Read the model definition and answer for the solid it produces. Units are mm, in the model's axes. Face numbers are marked on the shaded views. Coordinates: 2 decimals unless noted, no trailing zeros. Order: outer loops, then holes, each group sorted by start corner. A loop starts at its lowest first (then second) coordinate and runs counter-clockwise, first axis right, second up. Notation, with made-up numbers: (3, 75) -> (24, 75) arc R17 cw to (24, 105) -> close; hole circle Ø11 at (-39, 19). An arc over 180 degrees is marked (long way). Answer as a JSON object with one key per item and string values. Group by question number.
1) Section A-A on x = -48.75 is taken. Determine the outline of the cut face in (y, z).
2) Given pin 1 (1.5 mm diameter, centred on x = -51.5, y = 25.5, fed in from +Z); pin 2 (1.1 mm diameter, centred on y = 27.5, z = 3, fed in from +X); pin 3 (2 mm diameter, centred on y = 28, z = 4.5, fed in from -X), each flat-ended and moving along its own axis, determine where each tip first touches the part or whether it passes through.
3) Determine the mould class of the marked faces 1, 2, 3 and 4 for opening direction X: released by +X, released by -X, zero draft, split by the parting line, or undercut.
4) Consider L1, parallel to X at y = 26.75, z = 2.85; L2, parallel to Z at x = -50, y = 29.5; L3, parallel to X at y = 27.25, z = 0.9. Determine where each line is inside the solid, lowest interval first.
5) Section C-C on z = 3.15 is taken. Determine the outline of the cut face in (x, y), and give its area (3 significant figures).
6) Section D-D on x = -50 is taken. Determine the outline of the cut face in (y, z), and give its area (3 significant figures).
7) Section B-B on y = 24.75 is taken. Determine the outline of the cut face in (x, z).
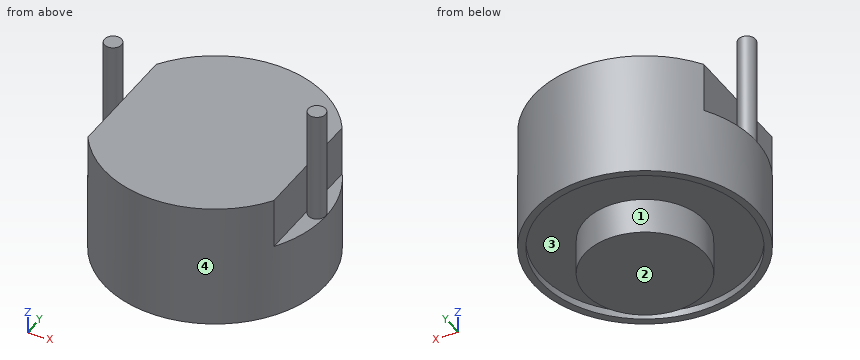
from build123d import *

# Parameters (mm, degrees)
SKETCH1_R            = 3.1
BOSS_EXTRUDE1_DEPTH  = 3.5
CUT_EXTRUDE1_START   = -1.4
CUT_EXTRUDE1_DEPTH   = 1.4
SKETCH4_R            = 0.24
BOSS_EXTRUDE23_DEPTH = 3.1
SKETCH5_R            = 0.24
BOSS_EXTRUDE24_DEPTH = 3.1
SKETCH6_R            = 2.9
CUT_EXTRUDE3_DEPTH   = 0.2
SKETCH7_R            = 1.675
BOSS_EXTRUDE25_DEPTH = 1


with BuildPart() as part:
    # Sketch1 → Boss-Extrude1 (new body)
    with BuildSketch(Plane.XY):
        with Locations((-49.1532488, 27.163637495)):
            Circle(SKETCH1_R)
    extrude(amount=BOSS_EXTRUDE1_DEPTH)

    # Sketch2 → Cut-Extrude1 (cut)
    with BuildSketch(Plane.XY.offset(3.5).offset(CUT_EXTRUDE1_START)):
        with BuildLine():
            Line((-51.7532488, 27.163637495), (-51.7532488, 28.851831796))
            ThreePointArc((-51.7532488, 28.851831796), (-52.2532488, 27.163637495), (-51.7532488, 25.475443193))
            Line((-51.7532488, 25.475443193), (-51.7532488, 27.163637495))
        make_face()
        with BuildLine():
            Line((-46.5532488, 27.163637495), (-46.5532488, 25.475443193))
            ThreePointArc((-46.5532488, 25.475443193), (-46.0532488, 27.163637495), (-46.5532488, 28.851831796))
            Line((-46.5532488, 28.851831796), (-46.5532488, 27.163637495))
        make_face()
    extrude(amount=CUT_EXTRUDE1_DEPTH, mode=Mode.SUBTRACT)

    # Sketch4 → Boss-Extrude23 (add)
    with BuildSketch(Plane.XY.offset(2.1)):
        with Locations((-46.3032488, 27.163637495)):
            Circle(SKETCH4_R)
    extrude(amount=BOSS_EXTRUDE23_DEPTH)

    # Sketch5 → Boss-Extrude24 (add)
    with BuildSketch(Plane.XY.offset(2.1)):
        with Locations((-52.0032488, 27.163637495)):
            Circle(SKETCH5_R)
    extrude(amount=BOSS_EXTRUDE24_DEPTH)

    # Sketch6 → Cut-Extrude3 (cut)
    with BuildSketch(Plane(origin=(0, 0, 0), x_dir=(-1, 0, 0), z_dir=(0, 0, -1))):
        with Locations((49.1532488, 27.163637495)):
            Circle(SKETCH6_R)
    extrude(amount=-CUT_EXTRUDE3_DEPTH, mode=Mode.SUBTRACT)

    # Sketch7 → Boss-Extrude25 (add)
    with BuildSketch(Plane(origin=(0, 0, 0.2), x_dir=(-1, 0, 0), z_dir=(0, 0, -1))):
        with Locations((49.1532488, 27.163637495)):
            Circle(SKETCH7_R)
    extrude(amount=BOSS_EXTRUDE25_DEPTH)


solid = part.part
Worked answers:
{
 "1": {"outline": "(24.09, 0) -> (24.29, 0) -> (24.29, 0.2) -> (25.54, 0.2) -> (25.54, -0.8) -> (28.79, -0.8) -> (28.79, 0.2) -> (30.04, 0.2) -> (30.04, 0) -> (30.24, 0) -> (30.24, 3.5) -> (24.09, 3.5) -> close"},
 "2": {"pin 1": "stops at z = 3.5", "pin 2": "stops at x = -46.06", "pin 3": "stops at x = -52.24"},
 "3": {"face 1": "undercut", "face 2": "zero draft", "face 3": "undercut", "face 4": "split by the parting line"},
 "4": {"L1": "x = -51.75 to -46.55", "L2": "z = 0.2 to 3.5", "L3": "x = -52.25 to -46.05"},
 "5": {"outline": "circle Ø0.48 at (-52, 27.16); (-51.75, 25.48) arc R3.1 ccw to (-46.55, 25.48) -> (-46.55, 28.85) arc R3.1 ccw to (-51.75, 28.85) -> close; circle Ø0.48 at (-46.3, 27.16)", "area": "28.3 mm²"},
 "6": {"outline": "(24.18, 0) -> (24.39, 0) -> (24.39, 0.2) -> (25.72, 0.2) -> (25.72, -0.8) -> (28.61, -0.8) -> (28.61, 0.2) -> (29.94, 0.2) -> (29.94, 0) -> (30.15, 0) -> (30.15, 3.5) -> (24.18, 3.5) -> close", "area": "22.7 mm²"},
 "7": {"outline": "(-51.1, 0) -> (-50.76, 0) -> (-50.76, 0.2) -> (-47.55, 0.2) -> (-47.55, 0) -> (-47.21, 0) -> (-47.21, 3.5) -> (-51.1, 3.5) -> close"}
}
